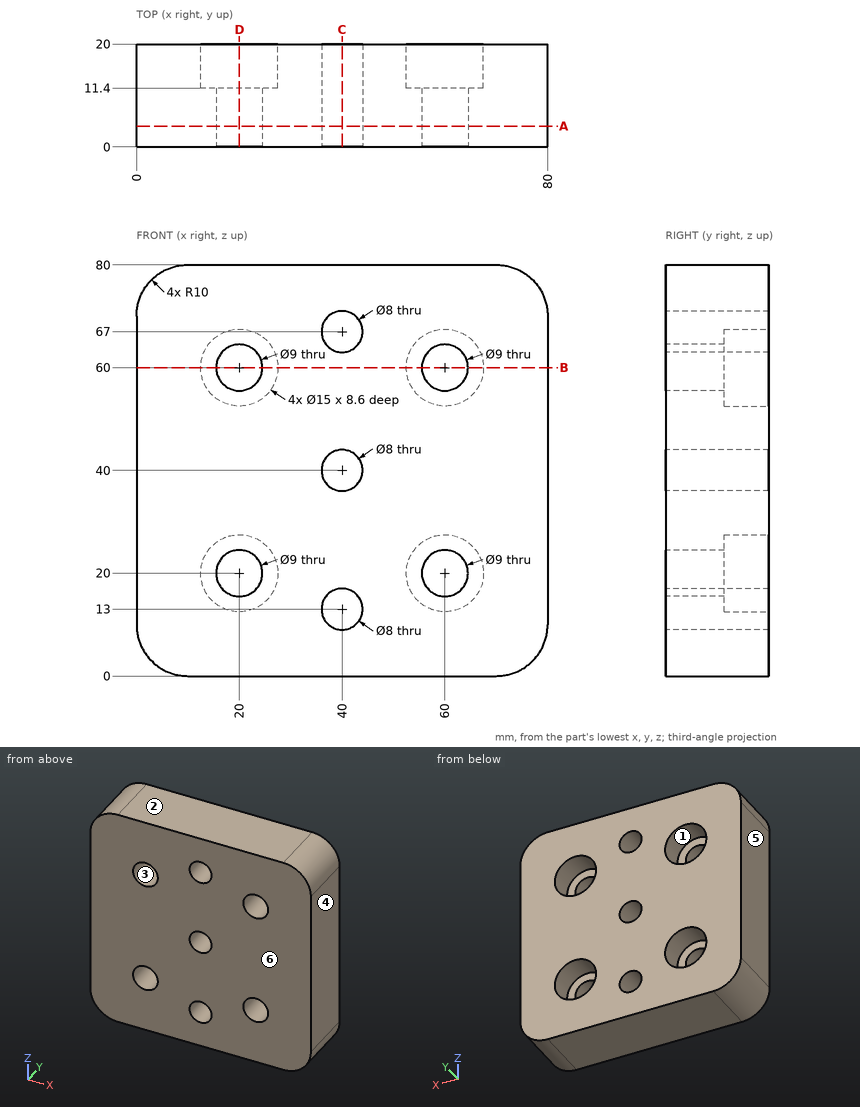
For this review, use the dimensioned drawing (mm, ordinates from the lowest corner) and the shaded views. A direction names the side the tool comes from. Give positions to 0.01 mm unless a question says otherwise; leave off trailing zeros. Loops run counter-clockwise (first coordinate to the right, second up) from the corner with the lowest first, then second, coordinate; pieces in that order, holes last. Notation, with made-up numbers: (-17, 4.5) -> (-7, 4.5) arc R16 cw to (-7, 31.5) -> close; hole circle Ø3 at (-16.75, -33.75). An arc over 180 degrees is marked (long way). One line per question, with ' | ' between items. Start each with the question number.
(1) For the marked faces 1 and 2, list the 3-axis set-ups (+Z, -Z, +X, -X, +Y, -Y) from which the entire face can be reached by the end or side of a thin tool; tool diameter is ignored.
(2) Insertion check: P1, Ø11.5, axis at x = 60, z = 20, coming from the +Y side. The pin has a flat end and moves straight along its axis. Give the tip position at first contact, or say it passes through.
(3) We need section B-B (z = 60). State the section outline as (x, y) points, and give its area (3 significant figures).
(4) We need section A-A (y = 4). State the section outline as (x, z) points.
(5) We need section C-C (x = 40). State the section outline as (y, z) points.
(6) For line 1 (Z direction, x = 20, y = 17.25); line 2 (Z direction, x = 40, y = 5), list the stretches that pass through material, from the lowest coordinate up.
(7) Draft analysis for pull direction X (two halves, no side actions). For the marked faces 3, 4, 5 and 6, state which applies: +X half, -X half, draft (parallel to the pull), parting line (faces both ways), or undercut.
(8) We need section D-D (x = 20). State the section outline as (y, z) points.
The answers:
1) face 1: +Y | face 2: +Z, +X, -X, +Y, -Y
2) P1: stops at y = 11.4
3) outline: (0, 0) -> (15.5, 0) -> (15.5, 11.4) -> (12.5, 11.4) -> (12.5, 20) -> (0, 20) -> close; (24.5, 0) -> (55.5, 0) -> (55.5, 11.4) -> (52.5, 11.4) -> (52.5, 20) -> (27.5, 20) -> (27.5, 11.4) -> (24.5, 11.4) -> close; (64.5, 0) -> (80, 0) -> (80, 20) -> (67.5, 20) -> (67.5, 11.4) -> (64.5, 11.4) -> close | area: 1,140 mm^2
4) outline: (0, 10) arc R10 ccw to (10, 0) -> (70, 0) arc R10 ccw to (80, 10) -> (80, 70) arc R10 ccw to (70, 80) -> (10, 80) arc R10 ccw to (0, 70) -> close; hole circle Ø9 at (20, 20); hole circle Ø9 at (20, 60); hole circle Ø8 at (40, 13); hole circle Ø8 at (40, 40); hole circle Ø8 at (40, 67); hole circle Ø9 at (60, 20); hole circle Ø9 at (60, 60)
5) outline: (0, 0) -> (20, 0) -> (20, 9) -> (0, 9) -> close; (0, 17) -> (20, 17) -> (20, 36) -> (0, 36) -> close; (0, 44) -> (20, 44) -> (20, 63) -> (0, 63) -> close; (0, 71) -> (20, 71) -> (20, 80) -> (0, 80) -> close
6) line 1: z = 0 to 12.5, 27.5 to 52.5, 67.5 to 80 | line 2: z = 0 to 9, 17 to 36, 44 to 63, 71 to 80
7) face 3: undercut | face 4: +X half | face 5: -X half | face 6: draft
8) outline: (0, 0) -> (20, 0) -> (20, 12.5) -> (11.4, 12.5) -> (11.4, 15.5) -> (0, 15.5) -> close; (0, 24.5) -> (11.4, 24.5) -> (11.4, 27.5) -> (20, 27.5) -> (20, 52.5) -> (11.4, 52.5) -> (11.4, 55.5) -> (0, 55.5) -> close; (0, 64.5) -> (11.4, 64.5) -> (11.4, 67.5) -> (20, 67.5) -> (20, 80) -> (0, 80) -> close
